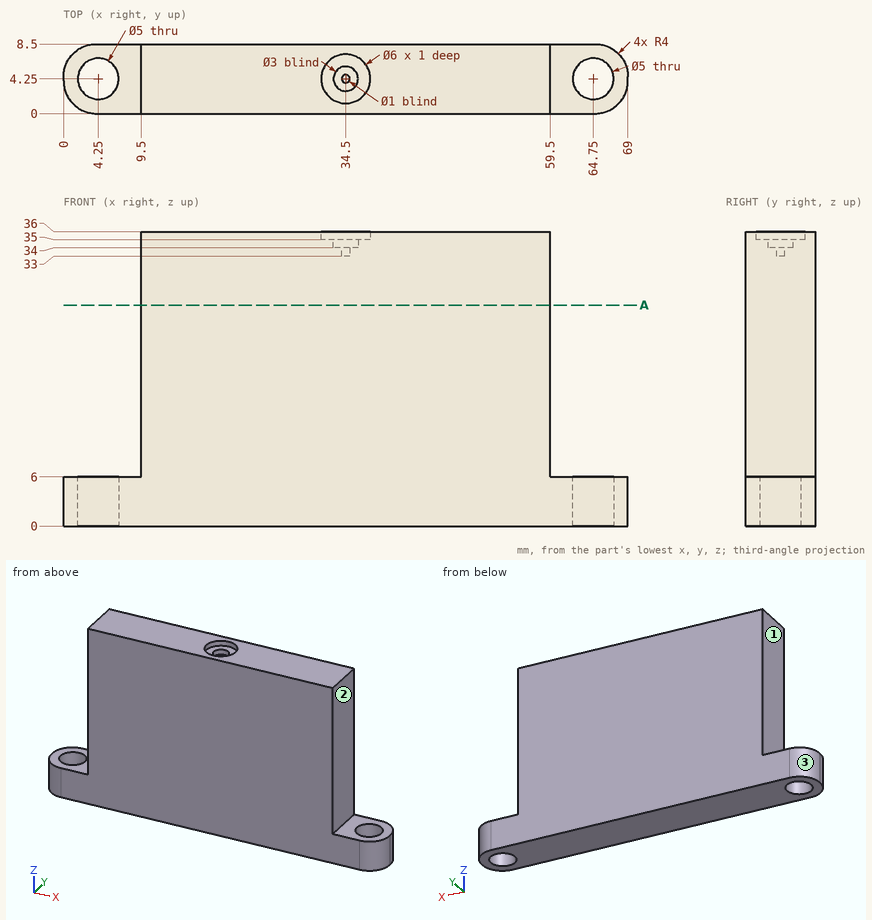
Job drawing, mm, ordinate dimensions from the low corner. One solid piece. A direction names the side the tool comes from. Give positions to 0.01 mm unless a question says otherwise; leave off trailing zeros. Order: outer loops, then holes, each group sorted by start corner. A loop starts at its lowest first (then second) coordinate and runs counter-clockwise, first axis right, second up. Notation, with made-up numbers: (-23, 54) - (2, 54) arc R10 ccw to (2, 65) - close; hole circle Ø1 at (4, 34). An arc over 180 degrees is marked (long way). One line per question, with ' | ' between items.
1. Drop flat-ended pins along their axis: P1, Ø5, axis at y = 2.5, z = 19.5, coming from the +X side; P2, Ø1.5, axis at x = 33.5, y = 4, coming from the +Z side; P3, Ø4, axis at y = 3, z = 14.5, coming from the -X side. Give the stop position or say it passes through.
Filled in:
P1: x = 59.5 | P2: z = 35 | P3: x = 9.5
2. Drill centre lines: probe 1 along X at (y, z) = (2.5, 2); probe 2 along Y at (x, z) = (4, 3); probe 3 along Y at (x, z) = (34.5, 34.2). Where is each one in solid material? Low to high.
Filled in:
probe 1: 0.29 to 2.46, 6.04 to 62.96, 66.54 to 68.71 | probe 2: 0 to 1.76, 6.74 to 8.5 | probe 3: 0 to 2.75, 5.75 to 8.5
3. Band-saw the part on A-A on z = 27. List the corners of the cut face in (x, y).
Filled in:
outline: (9.5, 0) - (59.5, 0) - (59.5, 8.5) - (9.5, 8.5) - close
4. Which spindle directions (+Z, -Z, +X, -X, +Y, -Y) get a long thin tool onto all of the face, cutting with end or side? Do the marked faces 1, 2 and 3. Say none if no direction does.
Filled in:
face 1: +Z, -X, +Y, -Y | face 2: +Z, +X, +Y, -Y | face 3: +Z, -Z, -X, +Y
